Input: part model. Units: mm. Frame: model coordinates. Face numbers are marked on the shaded views. A direction names the side the tool comes from. Coordinates: 2 decimals unless noted, no trailing zeros. Order: outer loops, then holes, each group sorted by start corner. A loop starts at its lowest first (then second) coordinate and runs counter-clockwise, first axis right, second up.
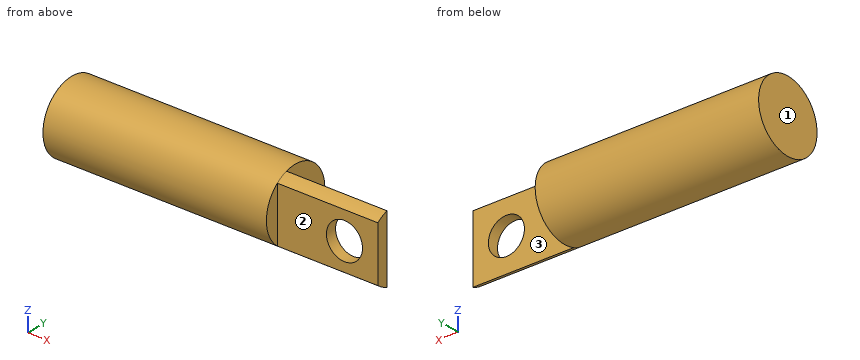
Autodesk Inventor part; units mm, degrees
ref_plane "YZ Plane" through (0, 0, 0) normal (1, 0, 0) x (0, 1, 0)
ref_plane "XZ Plane" through (0, 0, 0) normal (0, 1, 0) x (-1, 0, 0)
ref_plane "XY Plane" through (0, 0, 0) normal (0, 0, 1) x (1, 0, 0)
sketch "Sketch1" plane through (0, 0, 0) normal (1, 0, 0) x (0, 1, 0)
  circle A0 centre (0, 0) radius 8.001
  dimension "d0" = 16.002
extrude "Extrusion1" add sketch "Sketch1" along normal blind 50.8
sketch "Sketch2" plane through (50.8, 0, 0) normal (1, 0, 0) x (0, 0, -1)
  line L0 (-6.2432, -5.0038) -> (6.2432, -5.0038)
  line L1 (-7.5991, -2.5038) -> (7.5991, -2.5038)
  arc A0 (6.2432, -5.0038) -> (7.5991, -2.5038) centre (0, 0) ccw
  arc A1 (-7.5991, -2.5038) -> (-6.2432, -5.0038) centre (0, 0) ccw
  circle A2 centre (0, 0) radius 8.001
  point P0 (7.0332, -3.8145)
  point P1 (-7.0332, -3.8145)
  dimension "d3" = 5.0038
  dimension "d4" = 2.5
extrude "Extrusion2" add sketch "Sketch2" along normal blind 22.86 contours A1 L1 A0 L0
sketch "Sketch3" plane through (50.8, -2.5038, 7.5991) normal (0, 1, 0) x (1, 0, 0)
  circle A0 centre (15.2654, 7.5991) radius 4.1021
  line L0 (0, 15.1983) -> (22.86, 15.1983)
  line L1 (0, 0) -> (22.86, 0)
  line L2 (0, 0) -> (0, 15.1983)
  point P0 (-50.8, 7.5991)
  dimension "d8" = 8.2042
  dimension "d9" = 7.5991
  dimension "d10" = 15.1983
  dimension "d13" = 15.2654
extrude "Extrusion3" cut sketch "Sketch3" against normal blind 15.0114
equation "\"d9\" = 0.5 * d10"
properties part number "Ring Connector model 4"
Item 1: Pin query (flat end, axial travel): pin 1 Ø6 at (x, z) = (64, 1.5) entering from -Y; pin 2 Ø2 at (x, y) = (63, -4.5) entering from -Z; pin 3 Ø7.5 at (x, z) = (61, 1) entering from +Y. Return the tip coordinate at first contact, or that it passes through.
Response values:
pin 1: stops at y = -5
pin 2: stops at z = -7.19
pin 3: stops at y = -2.5
Item 2: Access query for the marked faces 1, 2 and 3. Directions: +Z, -Z, +X, -X, +Y, -Y. A direction counts if a zero-diameter tool reaches every point of the face in a straight line with its end or side. Return the directions, or none.
Response values:
face 1: +Z, -Z, -X, +Y, -Y
face 2: +Z, -Z, +X, -Y
face 3: +Z, -Z, +X, +Y
Item 3: Cut plane D-D on y = 0. Return loops of the section in (x, z), then the cut area to 3 significant figures.
Response values:
outline: (0, -8) - (50.8, -8) - (50.8, 8) - (0, 8) - close
area: 813 mm2
Item 4: Cut plane A-A on z = 0. Return loops of the section in (x, y).
Response values:
outline: (0, -8) - (50.8, -8) - (50.8, -5) - (61.96, -5) - (61.96, -2.5) - (50.8, -2.5) - (50.8, 8) - (0, 8) - close; (70.17, -5) - (73.66, -5) - (73.66, -2.5) - (70.17, -2.5) - close
Item 5: Cut plane C-C on y = -3.25. Return loops of the section in (x, z), then the cut area to 3 significant figures.
Response values:
outline: (0, -7.31) - (73.66, -7.31) - (73.66, 7.31) - (0, 7.31) - close; hole circle Ø8.2 at (66.07, 0)
area: 1,020 mm2
Item 6: Cut plane B-B on x = 63.5. Return loops of the section in (y, z), then the cut area to 3 significant figures.
Response values:
outline: (-5, -6.24) arc R8 ccw to (-2.5, -7.6) - (-2.5, -3.2) - (-5, -3.2) - close; (-5, 3.2) - (-2.5, 3.2) - (-2.5, 7.6) arc R8 ccw to (-5, 6.24) - close
area: 19.1 mm2
Item 7: Ray query, probe 1 along X at (y, z) = (-3.7, 0); probe 2 along X at (y, z) = (1.5, -5.5); probe 3 along Y at (x, z) = (57.5, -2.25). Return the intervals inside material, ascending.
Response values:
probe 1: x = 0 to 61.96, 70.17 to 73.66
probe 2: x = 0 to 50.8
probe 3: y = -5 to -2.5
